```python
from build123d import *

# Parameters (mm, degrees)
SKETCH_1_R          = 2.1
SKETCH_1_R_2        = 15.5
SKETCH_1_R_3        = 9.53
EXTRUDE_1_DEPTH     = 4
SKETCH_2_R          = 2
CUT_EXTRUDE_1_DEPTH = 10
EXTRUDE_2_DEPTH     = 4


with BuildPart() as part:
    # 草图1 → 凸台-拉伸1 (new body)
    with BuildSketch(Plane.XY):
        with BuildLine():
            ThreePointArc((-1.457142857, 39.854285714), (-41.457142857, -0.145714286), (-1.457142857, -40.145714286))
            Line((-1.457142857, -40.145714286), (348.542857143, -40.145714286))
            ThreePointArc((348.542857143, -40.145714286), (388.542857143, -0.145714286), (348.542857143, 39.854285714))
            Line((348.542857143, 39.854285714), (14.042857143, 39.854285714))
            Line((14.042857143, 39.854285714), (-1.457142857, 39.854285714))
        make_face()
        with Locations((-1.457142857, -23.895714286)):
            Circle(SKETCH_1_R, mode=Mode.SUBTRACT)
        with Locations((-20.942714442, -11.395714286)):
            Circle(SKETCH_1_R, mode=Mode.SUBTRACT)
        with Locations((18.028428728, -11.395714286)):
            Circle(SKETCH_1_R, mode=Mode.SUBTRACT)
        with Locations((-1.457142857, -0.145714286)):
            Circle(SKETCH_1_R_2, mode=Mode.SUBTRACT)
        with Locations((348.542857143, -0.145714286)):
            Circle(SKETCH_1_R_3, mode=Mode.SUBTRACT)
        with Locations((-22.025246197, 11.729285714)):
            Circle(SKETCH_1_R, mode=Mode.SUBTRACT)
        with Locations((19.110960483, 11.729285714)):
            Circle(SKETCH_1_R, mode=Mode.SUBTRACT)
        with Locations((-1.457142857, 22.354285714)):
            Circle(SKETCH_1_R, mode=Mode.SUBTRACT)
    extrude(amount=EXTRUDE_1_DEPTH)

    # 草图2 → 切除-拉伸1 (cut)
    with BuildSketch(Plane(origin=(0, 0, 0), x_dir=(-1, 0, 0), z_dir=(0, 0, -1))):
        with Locations((-20, -35.145714286)):
            Circle(SKETCH_2_R)
        with Locations((-115, -35.145714286)):
            Circle(SKETCH_2_R)
        with Locations((-210, -35.145714286)):
            Circle(SKETCH_2_R)
        with Locations((-305, -35.145714286)):
            Circle(SKETCH_2_R)
        with Locations((-305, 34.854285714)):
            Circle(SKETCH_2_R)
        with Locations((-210, 34.854285714)):
            Circle(SKETCH_2_R)
        with Locations((-115, 34.854285714)):
            Circle(SKETCH_2_R)
        with Locations((-20, 34.854285714)):
            Circle(SKETCH_2_R)
        Polygon((-218, -27.145714286), (-280.656658604, -27.145714286), (-218, 19.022349949), align=None)
        Polygon((-234.343341396, 26.854285714), (-297, -19.31377852), (-297, 26.854285714), align=None)
        Polygon((-123, 26.854285714), (-123, -19.31377852), (-185.656658604, 26.854285714), align=None)
        Polygon((-202, -27.145714286), (-139.343341396, -27.145714286), (-202, 19.022349949), align=None)
        Polygon((-90.656658604, -27.145714286), (-28, 19.022349949), (-28, -27.145714286), align=None)
        Polygon((-107, -19.31377852), (-44.343341396, 26.854285714), (-107, 26.854285714), align=None)
    extrude(amount=-CUT_EXTRUDE_1_DEPTH, mode=Mode.SUBTRACT)

    # 草图3 → 凸台-拉伸2 (add)
    with BuildSketch(Plane(origin=(0, 0, 0), x_dir=(-1, 0, 0), z_dir=(0, 0, -1))):
        Polygon((1.457142857, 39.854285714), (35.608920787, 39.854285714), (41.457142857, 39.854285714), (41.457142857, -0.145714286), align=None)
    extrude(amount=-EXTRUDE_2_DEPTH)


solid = part.part
```
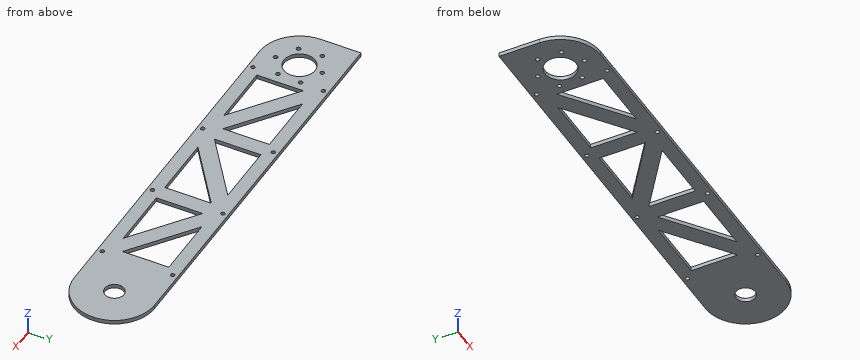
Build history of the part. All positions in model axes, mm. Give positions to 0.01 mm unless a question says otherwise; leave off trailing zeros. Loops run counter-clockwise (first coordinate to the right, second up) from the corner with the lowest first, then second, coordinate; pieces in that order, holes last.
1) Probe line 1 along Y through (x, z) = (210, 2.35); line 2 along X through (y, z) = (-27, 0.35); line 3 along Y through (x, z) = (244, 3.15). List the from-to ranges inside material, lowest first.
Values follow:
line 1: y = -40.15 to -37.15, -33.15 to 32.85, 36.85 to 39.85
line 2: x = -31.1 to 28, 90.46 to 139.54, 202 to 218, 280.46 to 378.19
line 3: y = -40.15 to -27.15, -0.14 to 19.74, 26.85 to 39.85
2) Band-saw the part on B-B on z = 1. State how many separate pieces and enclosed holes the cut face has, then the cut area to 3 significant figures.
Values follow:
separate pieces: 1
enclosed holes: 22
area: 23,500 mm2
3) Drop flat-ended pins along their axis: P1, Ø1.2, axis at y = 10.5, z = 2, coming from the +X side; P2, Ø3.5, axis at x = 210, y = 34.85, coming from the -Z side; P3, Ø1.5, axis at y = -30.5, z = 1, coming from the -X side; P4, Ø1.2, axis at y = 7, z = 2, coming from the +X side. Give the stop position or say it passes through.
Values follow:
P1: stops at x = 387.26
P2: passes through
P3: stops at x = -28.36
P4: stops at x = 388
4) Band-saw the part on A-A on x = 242. List the corners of the cut face in (y, z), then the cut area to 3 significant figures.
Values follow:
outline: (-40.15, 0) - (-27.15, 0) - (-27.15, 4) - (-40.15, 4) - close; (1.34, 0) - (21.21, 0) - (21.21, 4) - (1.34, 4) - close; (26.85, 0) - (39.85, 0) - (39.85, 4) - (26.85, 4) - close
area: 183 mm2
